Check sheet for the drawn part. Datum: minimum x, y, z corner. Units: mm. A direction names the side the tool comes from. Coordinates: 2 decimals unless noted, no trailing zeros. Loops run counter-clockwise (first coordinate to the right, second up) from the corner with the lowest first, then second, coordinate; pieces in that order, holes last. Notation, with made-up numbers: (-22, -16.75) - (19, -16.75) arc R18 ccw to (19, -6.75) - close; hole circle Ø9 at (1.5, 68.25). An arc over 180 degrees is marked (long way). Answer as a JSON object with one key per item and string values. Group by question number.
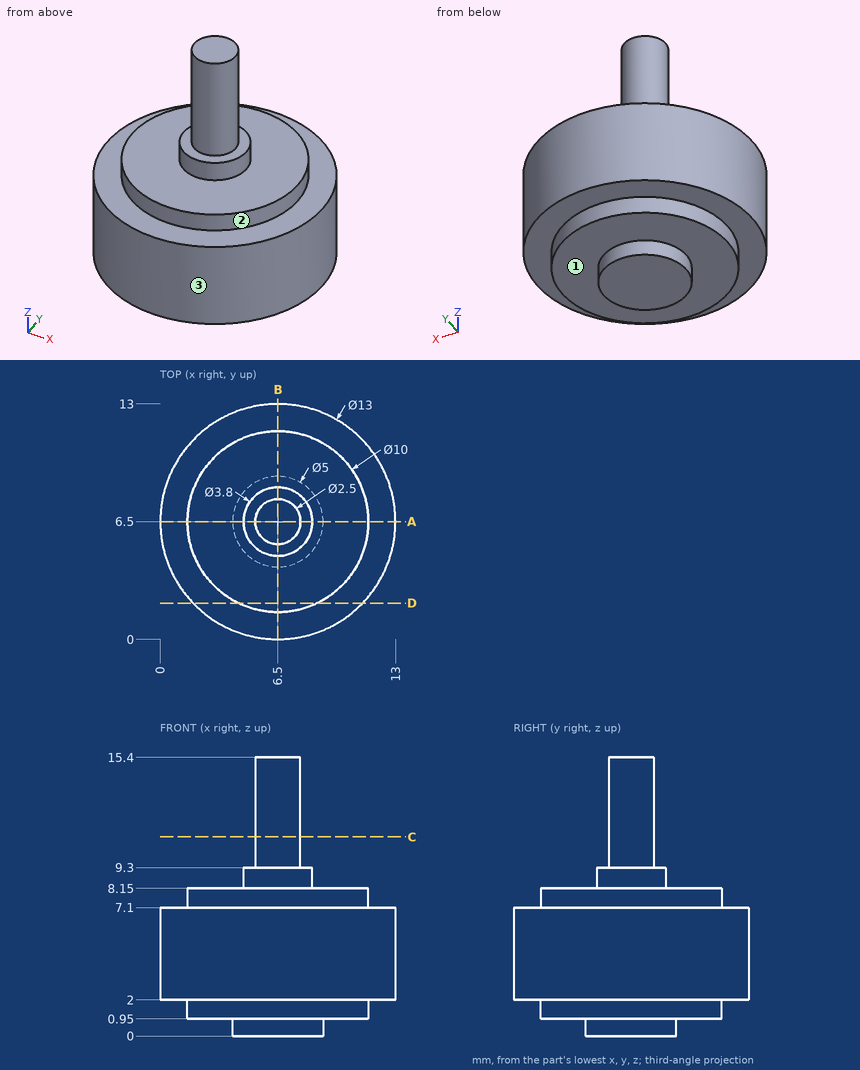
1. Gauge pin test, flat ends, axial feed: pin 1 (4 mm diameter, centred on x = 6, y = 1.5, fed in from +Z); pin 2 (6 mm diameter, centred on y = 7.5, z = 11, fed in from -X). Record the tip position at first contact, or that the pin passes through.
2. Sectioned sample at A-A on y = 6.5. Record the cut outline in (x, z).
3. Material ranges on line 1 (Z direction, x = 10.5, y = 7); line 2 (Z direction, x = 1.25, y = 5.25); line 3 (X direction, y = 7, z = 6.5), recorded low to high.
4. Access from +Z, -Z, +X, -X, +Y, -Y to the whole of each face (thin tool, end or side, straight path). Record for the marked faces 1, 2 and 3.
5. Sectioned sample at C-C on z = 11. Record the cut outline in (x, y), plus the area to 3 significant figures.
6. Sectioned sample at D-D on y = 2. Record the cut outline in (x, z), plus the area to 3 significant figures.
Answers follow:
{
 "1": {"pin 1": "stops at z = 8.15", "pin 2": "stops at x = 1.5"},
 "2": {"outline": "(0, 2) - (1.5, 2) - (1.5, 0.95) - (4, 0.95) - (4, 0) - (9, 0) - (9, 0.95) - (11.5, 0.95) - (11.5, 2) - (13, 2) - (13, 7.1) - (11.5, 7.1) - (11.5, 8.15) - (8.4, 8.15) - (8.4, 9.3) - (7.75, 9.3) - (7.75, 15.4) - (5.25, 15.4) - (5.25, 9.3) - (4.6, 9.3) - (4.6, 8.15) - (1.5, 8.15) - (1.5, 7.1) - (0, 7.1) - close"},
 "3": {"line 1": "z = 0.95 to 8.15", "line 2": "z = 2 to 7.1", "line 3": "x = 0.02 to 12.98"},
 "4": {"face 1": "-Z", "face 2": "+Z", "face 3": "+Z, -Z"},
 "5": {"outline": "circle Ø2.5 at (6.5, 6.5)", "area": "4.91 mm^2"},
 "6": {"outline": "(1.81, 2) - (4.32, 2) - (4.32, 0.95) - (8.68, 0.95) - (8.68, 2) - (11.19, 2) - (11.19, 7.1) - (8.68, 7.1) - (8.68, 8.15) - (4.32, 8.15) - (4.32, 7.1) - (1.81, 7.1) - close", "area": "57.0 mm^2"}
}
